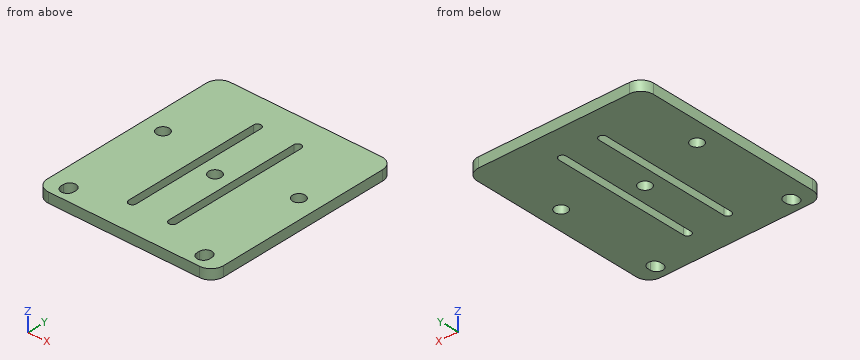
```python
from build123d import *

# Parameters (mm, degrees)
SKETCH4_W           = 70
SKETCH4_H           = 80
SKETCH4_R           = 2.5
BOSS_EXTRUDE2_DEPTH = 4
FILLET1_R           = 5
SKETCH6_R           = 2.5
CUT_EXTRUDE1_DEPTH  = 5


with BuildPart() as part:
    # Sketch4 → Boss-Extrude2 (new body)
    with BuildSketch(Plane.XY):
        Rectangle(SKETCH4_W, SKETCH4_H)
        with Locations((-27, 7)):
            Circle(SKETCH4_R, mode=Mode.SUBTRACT)
        with Locations((27, 7)):
            Circle(SKETCH4_R, mode=Mode.SUBTRACT)
        with BuildLine():
            Line((-24.5, -34), (-24.5, -35))
            ThreePointArc((-24.5, -35), (-27, -37.5), (-29.5, -35))
            Line((-29.5, -35), (-29.5, -34))
            ThreePointArc((-29.5, -34), (-27, -31.5), (-24.5, -34))
        make_face(mode=Mode.SUBTRACT)
        with BuildLine():
            Line((24.5, -34), (24.5, -35))
            ThreePointArc((24.5, -35), (27, -37.5), (29.5, -35))
            Line((29.5, -35), (29.5, -34))
            ThreePointArc((29.5, -34), (27, -31.5), (24.5, -34))
        make_face(mode=Mode.SUBTRACT)
    extrude(amount=BOSS_EXTRUDE2_DEPTH)

    # Fillet1
    fillet1_edges = [part.edges().sort_by_distance(p)[0] for p in [
        (35, -40, 2),
        (-35, -40, 2),
        (-35, 40, 2),
        (35, 40, 2),
    ]]
    fillet(fillet1_edges, radius=FILLET1_R)

    # Sketch6 → Cut-Extrude1 (cut, through all)
    with BuildSketch(Plane.XY.offset(4)):
        Circle(SKETCH6_R)
        with BuildLine():
            Line((-6.5, 27.5), (-6.5, -27.5))
            ThreePointArc((-6.5, -27.5), (-8, -29), (-9.5, -27.5))
            Line((-9.5, -27.5), (-9.5, 27.5))
            ThreePointArc((-9.5, 27.5), (-8, 29), (-6.5, 27.5))
        make_face()
        with BuildLine():
            Line((6.5, 27.5), (6.5, -27.5))
            ThreePointArc((6.5, -27.5), (8, -29), (9.5, -27.5))
            Line((9.5, -27.5), (9.5, 27.5))
            ThreePointArc((9.5, 27.5), (8, 29), (6.5, 27.5))
        make_face()
    extrude(amount=-CUT_EXTRUDE1_DEPTH, mode=Mode.SUBTRACT)


solid = part.part
```
CAD build for the part. Positions are in the model's coordinates, mm. Give positions to 0.01 mm unless a question says otherwise; leave off trailing zeros. Write each loop counter-clockwise with the first axis right and the second up, starting at its lowest first coordinate (ties: lowest second). Pieces come first, ordered by that corner, then holes. Notation, with made-up numbers: (72.5, 82) -> (103.5, 82) arc R13 ccw to (103.5, 101) -> close; hole circle Ø2 at (-7, 14.5). An arc over 180 degrees is marked (long way). Write each question's results on one line, items separated by ' | '.
1. Drop flat-ended pins along their axis: P1, Ø4.5, axis at x = -27, y = 7, coming from the -Z side; P2, Ø1, axis at x = 3, y = -13, coming from the -Z side. Give the stop position or say it passes through.
Geometry check:
P1: through | P2: z = 0
2. Cut at D-D, the plane z = 1.45. Write the cut outline in (x, y), then the cut area to 3 significant figures.
Geometry check:
outline: (-35, -35) arc R5 ccw to (-30, -40) -> (30, -40) arc R5 ccw to (35, -35) -> (35, 35) arc R5 ccw to (30, 40) -> (-30, 40) arc R5 ccw to (-35, 35) -> close; hole (-29.5, -35) arc R2.5 ccw to (-24.5, -35) -> (-24.5, -34) arc R2.5 ccw to (-29.5, -34) -> close; hole circle Ø5 at (-27, 7); hole (-9.5, -27.5) arc R1.5 ccw to (-6.5, -27.5) -> (-6.5, 27.5) arc R1.5 ccw to (-9.5, 27.5) -> close; hole circle Ø5 at (0, 0); hole (6.5, -27.5) arc R1.5 ccw to (9.5, -27.5) -> (9.5, 27.5) arc R1.5 ccw to (6.5, 27.5) -> close; hole (24.5, -35) arc R2.5 ccw to (29.5, -35) -> (29.5, -34) arc R2.5 ccw to (24.5, -34) -> close; hole circle Ø5 at (27, 7) | area: 5,130 mm²
3. Wall check: probe 1 along X at (y, z) = (-21.5, 3.05); probe 2 along Y at (x, z) = (27, 2.6); probe 3 along X at (y, z) = (6, 2.85). Give the ranges that are in metal, low to high. Write a range as [from, to].
Geometry check:
probe 1: [-35, -9.5], [-6.5, 6.5], [9.5, 35] | probe 2: [-40, -37.5], [-31.5, 4.5], [9.5, 40] | probe 3: [-35, -29.29], [-24.71, -9.5], [-6.5, 6.5], [9.5, 24.71], [29.29, 35]
4. Cut at B-B, the plane x = 27. Write the cut outline in (y, z), then the cut area to 3 significant figures.
Geometry check:
outline: (-40, 0) -> (-37.5, 0) -> (-37.5, 4) -> (-40, 4) -> close; (-31.5, 0) -> (4.5, 0) -> (4.5, 4) -> (-31.5, 4) -> close; (9.5, 0) -> (40, 0) -> (40, 4) -> (9.5, 4) -> close | area: 276 mm²
5. Cut at C-C, the plane y = -16. Write the cut outline in (x, z), then the cut area to 3 significant figures.
Geometry check:
outline: (-35, 0) -> (-9.5, 0) -> (-9.5, 4) -> (-35, 4) -> close; (-6.5, 0) -> (6.5, 0) -> (6.5, 4) -> (-6.5, 4) -> close; (9.5, 0) -> (35, 0) -> (35, 4) -> (9.5, 4) -> close | area: 256 mm²
6. Cut at A-A, the plane y = 7. Write the cut outline in (x, z), then the cut area to 3 significant figures.
Geometry check:
outline: (-35, 0) -> (-29.5, 0) -> (-29.5, 4) -> (-35, 4) -> close; (-24.5, 0) -> (-9.5, 0) -> (-9.5, 4) -> (-24.5, 4) -> close; (-6.5, 0) -> (6.5, 0) -> (6.5, 4) -> (-6.5, 4) -> close; (9.5, 0) -> (24.5, 0) -> (24.5, 4) -> (9.5, 4) -> close; (29.5, 0) -> (35, 0) -> (35, 4) -> (29.5, 4) -> close | area: 216 mm²
